The drawing under review shows one solid part. Ordinate dimensions are in mm from its lowest x, y, z. A direction names the side the tool comes from. Coordinates: 2 decimals unless noted, no trailing zeros. Order: outer loops, then holes, each group sorted by start corner. A loop starts at its lowest first (then second) coordinate and runs counter-clockwise, first axis right, second up. Notation, with made-up numbers: (82, 14.5) -> (139, 14.5) arc R15 cw to (139, 34.5) -> close; hole circle Ø11 at (-23, 50.5). An arc over 180 degrees is marked (long way). Use a Markdown table: item, result. Add a question column.
Q1. Add section C-C (y = 15.25). State the section outline as (x, z) points.
Q2. Add section B-B (x = 56.5). State the section outline as (y, z) points (1 decimal).
Q3. Insertion check: pin 1 (0.6 mm diameter, centred on x = 2, y = 10.5, fed in from +Z); pin 2 (3 mm diameter, centred on y = 7, z = 15, fed in from +X); pin 3 (8 mm diameter, centred on x = 34.5, z = 23, fed in from +Y). Each pin has a flat end and moves straight along its axis. Give the tip position at first contact, or say it passes through.
Q4. Machinability: for the marked faces 1, 2, 3 and 4, which of the approach directions +Z, -Z, +X, -X, +Y, -Y give a long, thin tool a straight path to every point of the face, cutting with its end or side? Answer none if there is none.
Q5. Add section D-D (z = 14). State the section outline as (x, y) points.
Q6. Wall thickness on probe 1 along Z at (x, y) = (13.5, 3.5); probe 2 along X at (y, z) = (2.5, 16); probe 3 along X at (y, z) = (3.5, 9) (1 decimal): over which ranges is each line inside the solid? List them lowest first.
Q7. Add section A-A (z = 3.5). State the section outline as (x, y) points.
Q8. The part is to be moulded in two halves that separate along X. For the marked faces 5, 6 and 7, say which applies: pulls with the +X half, pulls with the -X half, needs draft (parallel to the pull), parting line crosses it, or undercut.
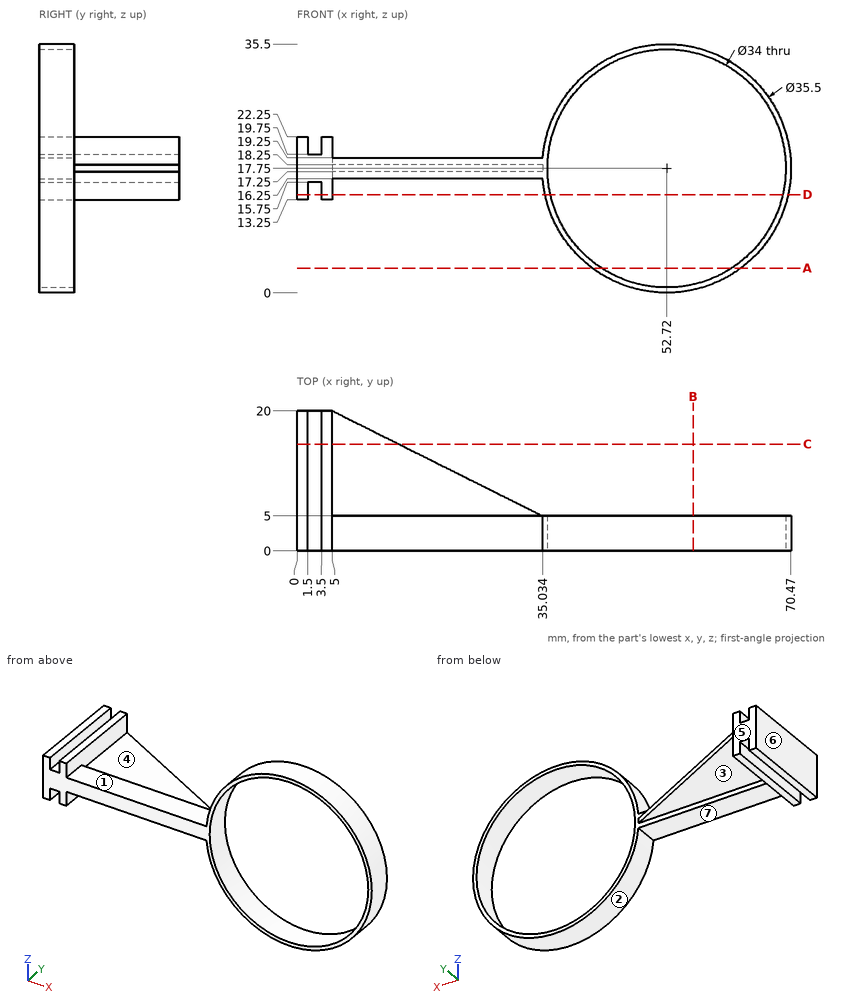
Established:
| question | item | result |
|---|---|---|
| 1 | outline | (0, 13.25) -> (1.5, 13.25) -> (1.5, 15.75) -> (3.5, 15.75) -> (3.5, 13.25) -> (5, 13.25) -> (5, 17.25) -> (14.51, 17.25) -> (14.51, 18.25) -> (5, 18.25) -> (5, 22.25) -> (3.5, 22.25) -> (3.5, 19.75) -> (1.5, 19.75) -> (1.5, 22.25) -> (0, 22.25) -> close |
| 2 | outline | (0, 0.4) -> (5, 0.4) -> (5, 1.2) -> (0, 1.2) -> close; (0, 34.3) -> (5, 34.3) -> (5, 35.1) -> (0, 35.1) -> close |
| 3 | pin 1 | z = 19.75 |
| 3 | pin 2 | x = 5 |
| 3 | pin 3 | y = 5 |
| 4 | face 1 | +Z, +Y, -Y |
| 4 | face 2 | +Y, -Y |
| 4 | face 3 | -Z, +X, +Y |
| 4 | face 4 | +Z, +X, +Y |
| 5 | outline | (0, 0) -> (1.5, 0) -> (1.5, 20) -> (0, 20) -> close; (3.5, 0) -> (5, 0) -> (5, 20) -> (3.5, 20) -> close; (35.37, 0) -> (36.14, 0) -> (36.14, 5) -> (35.37, 5) -> close; (69.3, 0) -> (70.07, 0) -> (70.07, 5) -> (69.3, 5) -> close |
| 6 | probe 1 | 16.25 to 19.25 |
| 6 | probe 2 | 0 to 5, 35.06 to 35.81, 69.63 to 70.38 |
| 6 | probe 3 | 37.3 to 38.1, 67.3 to 68.2 |
| 7 | outline | (42.14, 0) -> (43.45, 0) -> (43.45, 5) -> (42.14, 5) -> close; (61.99, 0) -> (63.3, 0) -> (63.3, 5) -> (61.99, 5) -> close |
| 8 | face 5 | needs draft |
| 8 | face 6 | pulls with the -X half |
| 8 | face 7 | undercut |
